Input: part model. Units: mm. Frame: model coordinates. Face numbers are marked on the shaded views. A direction names the side the tool comes from. Coordinates: 2 decimals unless noted, no trailing zeros. Write each loop counter-clockwise with the first axis right and the second up, starting at its lowest first coordinate (ties: lowest second). Pieces come first, ordered by that corner, then holes. Notation, with made-up numbers: (-15.75, 9.25) - (-7.75, 9.25) arc R11 ccw to (-7.75, 14.25) - close; hole circle Ø10 at (68.25, 8). An arc over 180 degrees is marked (long way). Use a Markdown table: item, result. Add a question column.
Q1. Section query D-D (z = 1.2). Return the cut outline in (x, y), then the cut area to 3 significant figures.
Q2. Section query B-B (x = 0). Return the cut outline in (y, z).
Q3. Mould query, pull axis X, two halves, no side actions, for the marked faces 1, 2, 3 and 4. Classes: released by +X, released by -X, zero draft, split by the parting line, or undercut.
Q4. Section query C-C (y = 4). Return the cut outline in (x, z), then the cut area to 3 significant figures.
Q5. Set-up query: the marked faces 5, 6 and 7. Return all of +Z, -Z, +X, -X, +Y, -Y with unobstructed straight access to the full face (end or side cutting, diameter ignored); none if empty.
Q6. Material intervals for probe 1 along Y at (x, z) = (0, 2.9); probe 2 along Y at (x, z) = (-1.25, 1.25); probe 3 along X at (y, z) = (1.5, 0.7), sorted ascending. Write a range as from..to.
Q7. Pin query (flat end, axial travel): P1, Ø1, axis at x = 1.5, y = -0.5, coming from the -Z side; P2, Ø0.7, axis at x = -0.5, y = -3.5, coming from the -Z side. Return the tip coordinate at first contact, or that it passes through.
Q8. Section query A-A (z = 4.3). Return the cut outline in (x, y), then the cut area to 3 significant figures.
Autodesk Inventor part; units mm, degrees
ref_plane "YZ Plane" through (0, 0, 0) normal (1, 0, 0) x (0, 1, 0)
ref_plane "XZ Plane" through (0, 0, 0) normal (0, 1, 0) x (-1, 0, 0)
ref_plane "XY Plane" through (0, 0, 0) normal (0, 0, 1) x (1, 0, 0)
sketch "Sketch1" plane through (0, 0, 0) normal (0, 0, 1) x (1, 0, 0)
  line L0 (-4, 8) -> (4, 8)
  line L1 (4, 8) -> (4, -8)
  line L2 (4, -8) -> (-4, -8)
  line L3 (-4, -8) -> (-4, 8)
  point P0 (0, 0)
  dimension "d0" = 8
  dimension "d1" = 16
  dimension "d2" = 4
  dimension "d3" = 8
extrude "Extrusion1" add sketch "Sketch1" along normal blind 3.2
shell "Shell1" thickness 1.5 removed faces 1 at (-1.3333, 2.6667, 0)
sketch "Sketch2" plane through (0, 0, 3.2) normal (0, 0, 1) x (1, 0, 0)
  circle A0 centre (0, -4) radius 2.5
  line L0 (4, 8) -> (4, -8)
  line L1 (4, -8) -> (-4, -8)
  dimension "d7" = 5
  dimension "d10" = 4
  dimension "d11" = 4
extrude "Extrusion2" add sketch "Sketch2" along normal blind 1.6
sketch "Sketch3" plane through (2.5, -6.5, 1.7) normal (0, 0, -1) x (-1, 0, 0)
  circle A0 centre (2.5, 2.5) radius 2.5
  circle A1 centre (2.5, 2.5) radius 1.2
  point P0 (2.5, 6.5)
  dimension "d18" = 2.4
extrude "Extrusion3" cut sketch "Sketch3" against normal blind 1.6 contours A1
pattern_linear "Rectangular Pattern1" count 2 spacing 8 along (0, 1, 0) of "Extrusion2", "Extrusion3"
sketch "Sketch4" plane through (2.5, -6.5, 1.7) normal (0, 0, -1) x (-1, 0, 0)
  circle A0 centre (2.5, 10.5) radius 1.2
  circle A1 centre (2.5, 2.5) radius 1.2
  line L0 (0, 13) -> (0, 0)
  line L1 (0, 0) -> (5, 0)
  circle A2 centre (6.5, 6.5) radius 3.15
  circle A3 centre (6.5, 6.5) radius 2.5
  point P0 (2.5, 6.5)
  dimension "d21" = 6.5
  dimension "d22" = 6.5
  dimension "d23" = 10.5
  dimension "d24" = 2.5
  dimension "d25" = 5
  dimension "d26" = 6.3
extrude "Extrusion4" [suppressed]
pattern_linear "Rectangular Pattern2" [suppressed]
equation "\"d0\" = 0.8 * WIDTH"
equation "\"d1\" = 0.8 * LENGTH"
equation "\"d4\" = HEIGHT"
equation "\"d21\" = 0.5 * d23 + 0.5 * d24"
equation "\"d22\" = d21"
equation "\"WIDTH\" = 1"
equation "\"HEIGHT\" = 3.2"
properties part number "3023" material "Steel"
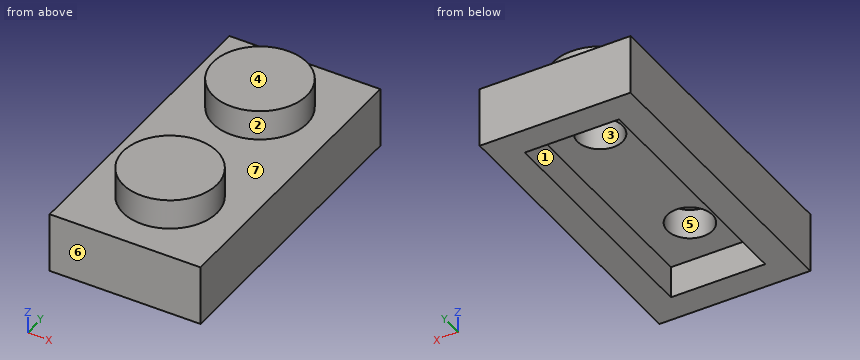
Values follow:
| question | item | result |
|---|---|---|
| 1 | outline | (-4, -8) - (4, -8) - (4, 8) - (-4, 8) - close; hole (-2.5, -6.5) - (2.5, -6.5) - (2.5, 6.5) - (-2.5, 6.5) - close |
| 1 | area | 63.0 mm2 |
| 2 | outline | (-8, 0) - (-6.5, 0) - (-6.5, 1.7) - (-5.2, 1.7) - (-5.2, 3.3) - (-2.8, 3.3) - (-2.8, 1.7) - (2.8, 1.7) - (2.8, 3.3) - (5.2, 3.3) - (5.2, 1.7) - (6.5, 1.7) - (6.5, 0) - (8, 0) - (8, 3.2) - (6.5, 3.2) - (6.5, 4.8) - (1.5, 4.8) - (1.5, 3.2) - (-1.5, 3.2) - (-1.5, 4.8) - (-6.5, 4.8) - (-6.5, 3.2) - (-8, 3.2) - close |
| 3 | face 1 | undercut |
| 3 | face 2 | split by the parting line |
| 3 | face 3 | undercut |
| 3 | face 4 | zero draft |
| 4 | outline | (-4, 0) - (-2.5, 0) - (-2.5, 1.7) - (-1.2, 1.7) - (-1.2, 3.3) - (1.2, 3.3) - (1.2, 1.7) - (2.5, 1.7) - (2.5, 0) - (4, 0) - (4, 3.2) - (2.5, 3.2) - (2.5, 4.8) - (-2.5, 4.8) - (-2.5, 3.2) - (-4, 3.2) - close |
| 4 | area | 21.3 mm2 |
| 5 | face 5 | -Z |
| 5 | face 6 | +Z, -Z, +X, -X, -Y |
| 5 | face 7 | +Z |
| 6 | probe 1 | -8..-5.2, -2.8..2.8, 5.2..8 |
| 6 | probe 2 | -8..-6.5, 6.5..8 |
| 6 | probe 3 | -4..-2.5, 2.5..4 |
| 7 | P1 | z = 1.7 |
| 7 | P2 | z = 3.3 |
| 8 | outline | circle Ø5 at (0, -4); circle Ø5 at (0, 4) |
| 8 | area | 39.3 mm2 |
